The listing builds one solid part. Answer for the finished solid, in the listing's coordinates (mm). A direction names the side the tool comes from. Coordinates: 2 decimals unless noted, no trailing zeros. Loops run counter-clockwise (first coordinate to the right, second up) from the corner with the lowest first, then second, coordinate; pieces in that order, holes last. Notation, with made-up numbers: (-12.5, 65) - (9.5, 65) arc R28 cw to (9.5, 89) - close; hole circle Ø3 at (79.25, -32). An arc over 180 degrees is marked (long way). Return JSON: item names as keys, results as strings. Group by question number.
1. Section D-D (x = 28) is taken. Write down the section's boundary in (y, z).
2. Find the intervals of material crossed by line 1 along X through (y, z) = (-46, 16); line 2 along X through (y, z) = (-16, -34); line 3 along X through (y, z) = (0, -31), in increasing order.
3. Section C-C (y = 0) is taken. State how many separate pieces and enclosed holes the cut face has, and give its area (3 significant figures).
4. Which of the six approach directions +Z, -Z, +X, -X, +Y, -Y give full straight-line access (tool end or side, diameter ignored) to faces 4 (the face through (10.01, 15.62, -3.47)), 5 (the face through (44.417, 0, -37)), 6 (the face through (32.743, 0.477, -26.759)), 7 (the face through (6.4, -55.4, -7.3))?
5. Each of these flat-tipped pins is pushed along its axis until it touches: P1, Ø3, axis at y = -24.5, z = 30, coming from the +X side; P2, Ø17.5, axis at y = 0, z = 0, coming from the -X side; P3, Ø2, axis at y = -4.5, z = -37, coming from the -X side; P4, Ø1, axis at x = 17, z = 3, coming from the -Y side. Where does it stop, or does it pass through?
6. Section A-A (x = 13) is taken. Write down the section's boundary in (y, z), and give its area (3 significant figures).
7. The mould has two halves that part along X. Classify faces 1 (the face through (37, 0, -35.56)), 2 (the face through (50.28, 13.91, -18.14)), 3 (the face through (48.608, -1, 24)): pulls with the +X half, pulls with the -X half, needs draft (parallel to the pull), parting line crosses it, or undercut.
8. Section B-B (z = -48.5) is taken. Write down the section's boundary in (x, y).
```python
from build123d import *

# Parameters (mm, degrees)
SKETCH3_W                         = 20.32
SKETCH3_H                         = 50.8
CUT_EXTRUDE1_DEPTH                = 2.54
F_1_8_0_125_DIAMETER_HOLE1_REACH  = 123.254
F_1_8_0_125_DIAMETER_HOLE1_BORE_R = 1.5875
FILLET2_R                         = 1.778
CHAMFER1_SIZE                     = 0.508


with BuildPart() as part:
    # Sketch1 → Revolve1 (revolve)
    with BuildSketch(Plane.XY, mode=Mode.PRIVATE) as revolve1_sk:
        Polygon((3.81, 55.88), (8.89, 55.88), (8.89, 38.1), (43.5280054, 38.1), (43.5280054, 55.88), (48.6080054, 55.88), (48.6080054, 22.86), (52.4180054, 22.86), (52.4180054, 17.78), (15.0800054, 17.78), (15.0800054, 16.002), (5.08, 16.002), (5.08, 11.079988), (0, 11.079988), (0, 22.86), (3.81, 22.86), align=None)
    revolve(revolve1_sk.sketch.rotate(Axis((0, 0, 0), (1, 0, 0)), 90), axis=Axis((0, 0, 0), (1, 0, 0)))

    # Sketch3 → Cut-Extrude1 (cut)
    with BuildSketch(Plane(origin=(0, 0, -38.1), x_dir=(-1, 0, 0), z_dir=(0, 0, -1))):
        with Locations((-34.2570054, 0)):
            Rectangle(SKETCH3_W, SKETCH3_H)
    extrude(amount=-CUT_EXTRUDE1_DEPTH, mode=Mode.SUBTRACT)

    # 1/8 (0.125) Diameter Hole1 bore → 1/8 (0.125) Diameter Hole1 (cut, up to next)
    with BuildSketch(Plane(origin=(0, 0, -38.1), x_dir=(-1, 0, 0), z_dir=(0, 0, -1)), mode=Mode.PRIVATE) as f_1_8_0_125_diameter_hole1_sk1:
        with Locations((-34.2570054, 0)):
            Circle(F_1_8_0_125_DIAMETER_HOLE1_BORE_R)
    f_1_8_0_125_diameter_hole1_tool1 = extrude(f_1_8_0_125_diameter_hole1_sk1.sketch, amount=-F_1_8_0_125_DIAMETER_HOLE1_REACH, mode=Mode.PRIVATE) & part.part
    add(f_1_8_0_125_diameter_hole1_tool1.solids().sort_by_distance((34.257005, 0, -38.1))[0], mode=Mode.SUBTRACT)

    # Fillet2
    fillet2_edges = [part.edges().sort_by_distance(p)[0] for p in [
        (8.89, 0, -38.1),
        (43.5280054, 37.459618258, 6.95607648),
    ]]
    fillet(fillet2_edges, radius=FILLET2_R)

    # Chamfer1
    chamfer1_edges = [part.edges().sort_by_distance(p)[0] for p in [
        (0, 0, -22.86),
        (0, 0, -11.079988),
        (52.4180054, 0, -17.78),
        (52.4180054, 0, -22.86),
    ]]
    chamfer(chamfer1_edges, length=CHAMFER1_SIZE)


solid = part.part
```
The answers:
{
 "1": {"outline": "(-13.68, -35.56) - (13.68, -35.56) arc R38.1 ccw (long way) to start; hole circle Ø35.56 at (0, 0)"},
 "2": {"line 1": "x = 3.81 to 8.89, 43.53 to 48.61", "line 2": "x = 3.81 to 48.61", "line 3": "x = 3.81 to 32.67, 35.84 to 48.61"},
 "3": {"separate pieces": "3", "enclosed holes": "0", "area": "2,260 mm2"},
 "4": {"face 4": "+X", "face 5": "none", "face 6": "-Z", "face 7": "+X, -X"},
 "5": {"P1": "stops at x = 48.61", "P2": "passes through", "P3": "stops at x = 3.81", "P4": "stops at y = -38.02"},
 "6": {"outline": "circle Ø76.2 at (0, 0); hole circle Ø32 at (0, 0)", "area": "3,760 mm2"},
 "7": {"face 1": "undercut", "face 2": "needs draft", "face 3": "pulls with the +X half"},
 "8": {"outline": "(3.81, -27.75) - (8.89, -27.75) - (8.89, 27.75) - (3.81, 27.75) - close; (43.53, -27.75) - (48.61, -27.75) - (48.61, 27.75) - (43.53, 27.75) - close"}
}
